Verification items for this drawing (mm, ordinates from the low corner). A direction names the side the tool comes from. Round coordinates to 2 decimals unless told otherwise and drop trailing zeros. Loops run counter-clockwise (first coordinate to the right, second up) from the corner with the lowest first, then second, coordinate; pieces in that order, holes last. Notation, with made-up numbers: M 76.5,-12 L 132.5,-12 A18 ccw 132.5,-1 Z; hole C -36.5,-32.75 d10. An arc over 180 degrees is marked long. One line per item, written item: value.
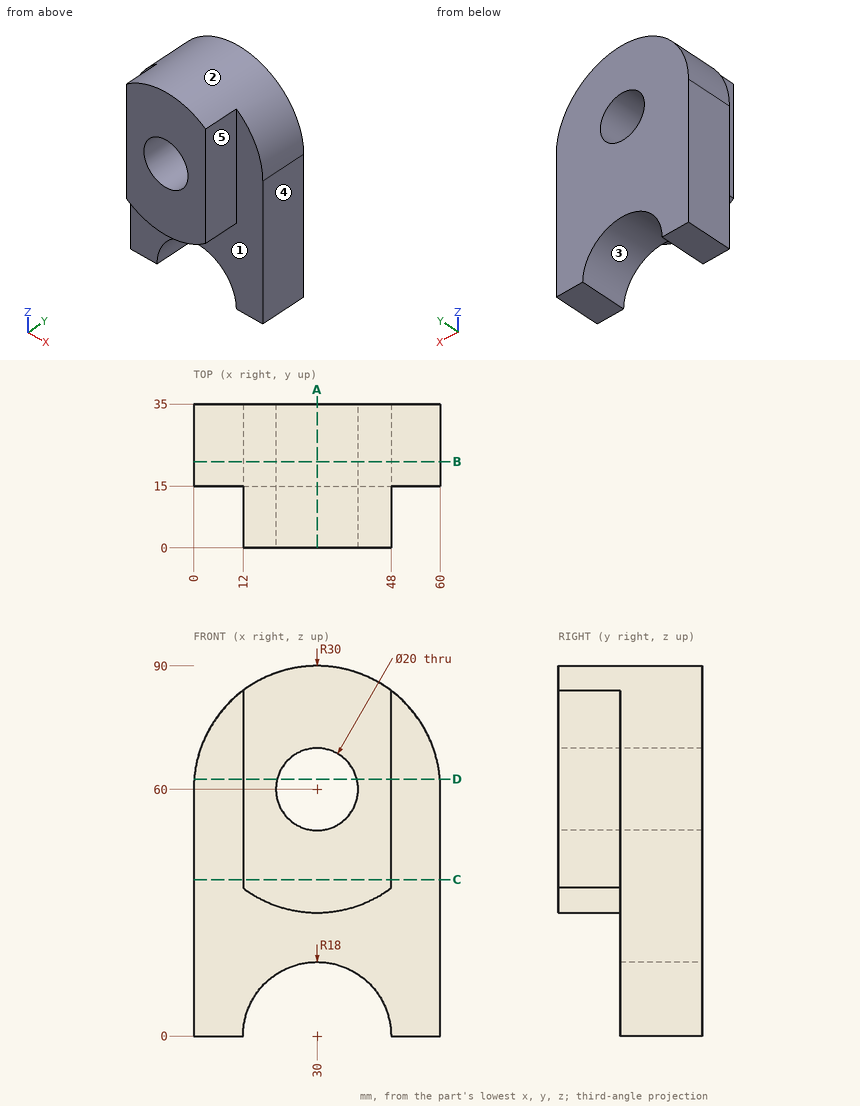
(1) Thickness scan on L1, parallel to Z at x = 30, y = 26; L2, parallel to X at y = 22, z = 53; L3, parallel to Y at x = 55.5, z = 40.5. Record the ranges inside material, lowest first. Write a range as from..to.
Completed:
L1: z = 18..50, 70..90
L2: x = 0..22.86, 37.14..60
L3: y = 15..35
(2) Sectioned sample at A-A on x = 30. Enter the section's corners in (y, z), and give its area (3 significant figures).
Completed:
outline: M 0,30 L 15,30 L 15,18 L 35,18 L 35,50 L 0,50 Z; M 0,70 L 35,70 L 35,90 L 0,90 Z
area: 1,640 mm^2
(3) Sectioned sample at D-D on z = 62.5. Enter the section's corners in (x, y), and give its area (3 significant figures).
Completed:
outline: M 0.1,15 L 12,15 L 12,0 L 20.32,0 L 20.32,35 L 0.1,35 Z; M 39.68,0 L 48,0 L 48,15 L 59.9,15 L 59.9,35 L 39.68,35 Z
area: 1,060 mm^2
(4) Sectioned sample at C-C on z = 38. Enter the section's corners in (x, y).
Completed:
outline: M 0,15 L 12,15 L 12,0 L 48,0 L 48,15 L 60,15 L 60,35 L 0,35 Z
(5) Tool access check on the marked faces 4 and 5. Record the directions out of +Z, -Z, +X, -X, +Y, -Y that give a thin tool (end or side, any length) a straight path to the whole face; none if there is none.
Completed:
face 4: +Z, -Z, +X, +Y, -Y
face 5: +Z, -Z, +X, -Y
(6) Sectioned sample at B-B on y = 21. Enter the section's corners in (x, z), and give its area (3 significant figures).
Completed:
outline: M 0,0 L 12,0 A18 cw 48,0 L 60,0 L 60,60 A30 ccw 0,60 Z; hole C 30,60 d20
area: 4,190 mm^2
(7) Mould release check, pull along X, two halves, no side actions. Record for the marked faces 1, 2 and 3: +X half, -X half, draft (parallel to the pull), parting line (faces both ways), or undercut.
Completed:
face 1: draft
face 2: parting line
face 3: undercut
(8) Depth check by flat-ended pin: pin 1 Ø12 at (y, z) = (11, 13.5) entering from -X; pin 2 Ø12 at (y, z) = (7.5, 49) entering from +X; pin 3 Ø10 at (x, y) = (37, 23.5) entering from -Z; pin 4 Ø4 at (x, y) = (18.5, 30) entering from -Z. Enter the tip coordinate at first touch or a pass-through.
Completed:
pin 1: stops at x = 0
pin 2: stops at x = 48
pin 3: stops at z = 13.42
pin 4: stops at z = 11.91
